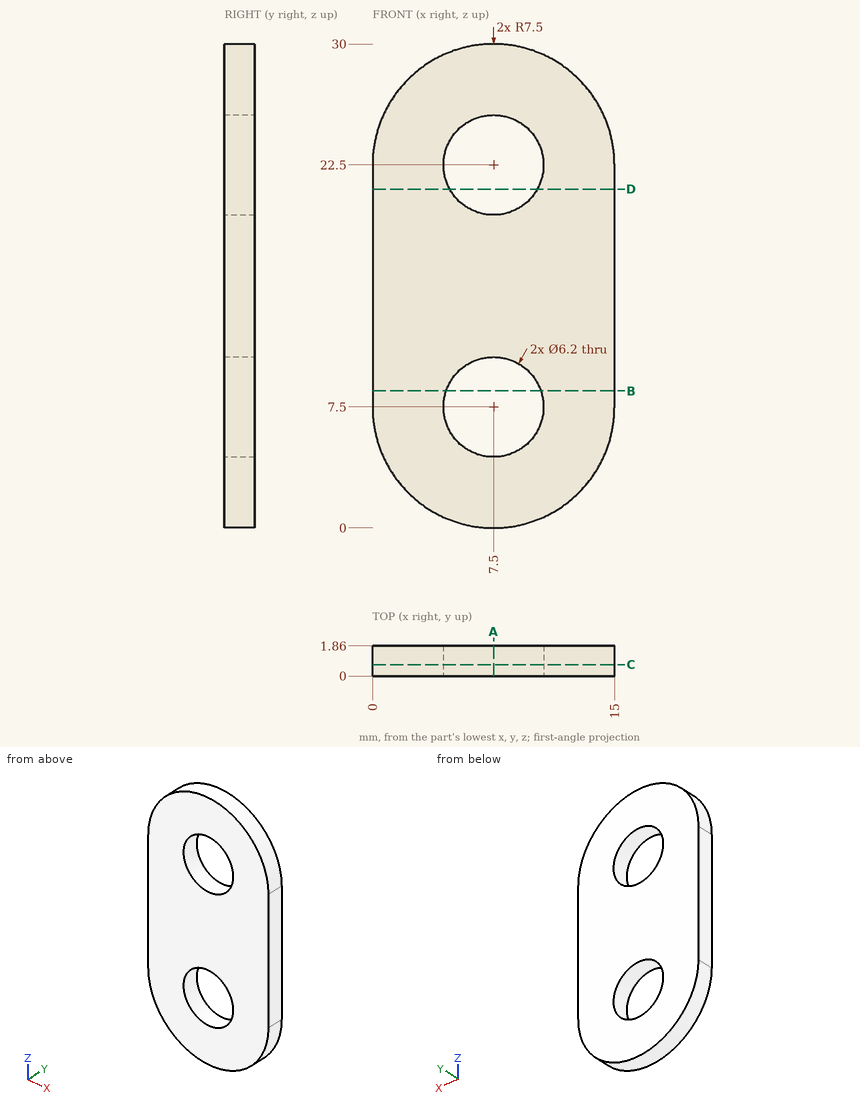
The drawing under review shows one solid part. Ordinate dimensions are in mm from its lowest x, y, z. Round coordinates to 2 decimals unless told otherwise and drop trailing zeros. Write each loop counter-clockwise with the first axis right and the second up, starting at its lowest first coordinate (ties: lowest second). Pieces come first, ordered by that corner, then holes. Notation, with made-up numbers: M 32,-30 L 80,-30 A26 ccw 80,-5 Z; hole C 29.5,-4.75 d7. An arc over 180 degrees is marked long. One line per item, written item: value. Start each with the question number.
(1) We need section D-D (z = 21). Give the boundary of the cut face in (x, y), and give its area (3 significant figures).
(2) We need section A-A (x = 7.5). Give the boundary of the cut face in (y, z), and give its area (3 significant figures).
(3) We need section C-C (y = 0.7). Give the boundary of the cut face in (x, z).
(4) We need section B-B (z = 8.5). Give the boundary of the cut face in (x, y).
(5) Wall thickness on line 1 (X direction, y = 0.55, z = 22.5); line 2 (Z direction, x = 9.5, y = 0.7); line 3 (Z direction, x = 8, y = 1.7): over which ranges is each line inside the solid? List them lowest first.
Result:
1. outline: M 0,0 L 4.79,0 L 4.79,1.86 L 0,1.86 Z; M 10.21,0 L 15,0 L 15,1.86 L 10.21,1.86 Z
1. area: 17.8 mm²
2. outline: M 0,0 L 1.86,0 L 1.86,4.4 L 0,4.4 Z; M 0,10.6 L 1.86,10.6 L 1.86,19.4 L 0,19.4 Z; M 0,25.6 L 1.86,25.6 L 1.86,30 L 0,30 Z
2. area: 32.7 mm²
3. outline: M 0,7.5 A7.5 ccw 15,7.5 L 15,22.5 A7.5 ccw 0,22.5 Z; hole C 7.5,7.5 d6.2; hole C 7.5,22.5 d6.2
4. outline: M 0,0 L 4.57,0 L 4.57,1.86 L 0,1.86 Z; M 10.43,0 L 15,0 L 15,1.86 L 10.43,1.86 Z
5. line 1: 0 to 4.4, 10.6 to 15
5. line 2: 0.27 to 5.13, 9.87 to 20.13, 24.87 to 29.73
5. line 3: 0.02 to 4.44, 10.56 to 19.44, 25.56 to 29.98
